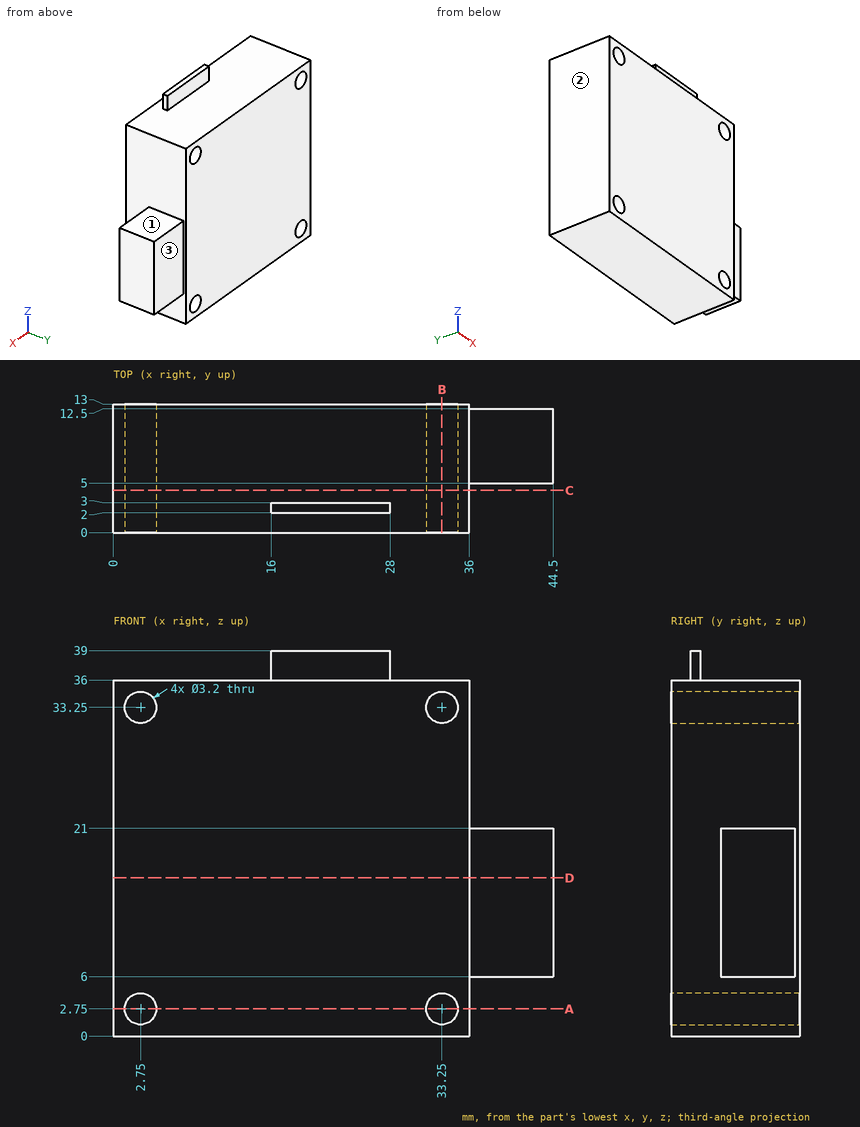
Study the drawing (mm; zero at the part's minimum x, y, z) and answer. A direction names the side the tool comes from. Coordinates: 2 decimals unless noted, no trailing zeros. Loops run counter-clockwise (first coordinate to the right, second up) from the corner with the lowest first, then second, coordinate; pieces in that order, holes last. Notation, with made-up numbers: M 8,-25 L 45,-25 A21 ccw 45,14 Z; hole C -38,39 d10. An arc over 180 degrees is marked long. Answer as a JSON object with one key per item and string values. Group by question number.
Item 1: Section D-D (z = 16) is taken. Write down the section's boundary in (x, y).
Item 2: Which of the six approach directions +Z, -Z, +X, -X, +Y, -Y give full straight-line access (tool end or side, diameter ignored) to the marked faces 1, 2 and 3?
Item 3: Each of these flat-tipped pins is pushed along its axis until it touches: P1, Ø4, axis at x = 10.5, y = 5.5, coming from the +Z side; P2, Ø1.1, axis at y = 2.5, z = 37, coming from the +X side; P3, Ø1.5, axis at y = 9.5, z = 5, coming from the +X side. Where does it stop, or does it pass through?
Item 4: Section B-B (x = 33.25) is taken. Write down the section's boundary in (y, z), and give its area (3 significant figures).
Item 5: Section C-C (y = 4.25) is taken. Write down the section's boundary in (x, z), and give its area (3 significant figures).
Item 6: Section A-A (z = 2.75) is taken. Write down the section's boundary in (x, y), and give its area (3 significant figures).
Item 7: Consider L1, parallel to X at y = 10.25, z = 33.25; L2, parallel to Z at x = 21, y = 12. Determine where each line is inside the solid, lowest interval first.
Solved:
{
 "1": {"outline": "M 0,0 L 36,0 L 36,5 L 44.5,5 L 44.5,12.5 L 36,12.5 L 36,13 L 0,13 Z"},
 "2": {"face 1": "+Z, +X, +Y, -Y", "face 2": "+Z, -Z, -X, +Y, -Y", "face 3": "+Z, -Z, +X, +Y"},
 "3": {"P1": "stops at z = 36", "P2": "stops at x = 28", "P3": "stops at x = 36"},
 "4": {"outline": "M 0,0 L 13,0 L 13,1.15 L 0,1.15 Z; M 0,4.35 L 13,4.35 L 13,31.65 L 0,31.65 Z; M 0,34.85 L 13,34.85 L 13,36 L 0,36 Z", "area": "385 mm2"},
 "5": {"outline": "M 0,0 L 36,0 L 36,36 L 0,36 Z; hole C 2.75,2.75 d3.2; hole C 2.75,33.25 d3.2; hole C 33.25,2.75 d3.2; hole C 33.25,33.25 d3.2", "area": "1,260 mm2"},
 "6": {"outline": "M 0,0 L 1.15,0 L 1.15,13 L 0,13 Z; M 4.35,0 L 31.65,0 L 31.65,13 L 4.35,13 Z; M 34.85,0 L 36,0 L 36,13 L 34.85,13 Z", "area": "385 mm2"},
 "7": {"L1": "x = 0 to 1.15, 4.35 to 31.65, 34.85 to 36", "L2": "z = 0 to 36"}
}
